```python
from build123d import *

# Parameters (mm, degrees)
F1_DEPTH = 20
F3_DEPTH = 20


with BuildPart() as f1:
    # F0 (on Top) → F1 (new body)
    with BuildSketch(Plane.XY):
        with BuildLine():
            ThreePointArc((-8.944425, -1.9), (0.955226, -9.093969), (9.144, 0))
            ThreePointArc((9.144, 0), (0.955226, 9.093969), (-8.944425, 1.9))
            ThreePointArc((-8.944425, 1.9), (-9.144, 0), (-8.944425, -1.9))
        make_face()
        with BuildLine():
            ThreePointArc((-8.944425, -1.9), (-9.144, 0), (-8.944425, 1.9))
            Line((-8.944425, 1.9), (-11.644, 1.9))
            Line((-11.644, 1.9), (-11.644, -1.9))
            Line((-11.644, -1.9), (-8.944425, -1.9))
        make_face()
    extrude(amount=F1_DEPTH)

    # F2 (on face) → F3 (cut, through all)
    with BuildSketch(Plane.XY.offset(20)):
        Polygon((6.6675, -3.849483), (6.6675, 3.849483), (0, 7.698966), (-6.6675, 3.849483), (-6.6675, -3.849483), (0, -7.698966), align=None)
    extrude(amount=-F3_DEPTH, mode=Mode.SUBTRACT)


solid = f1.part
```
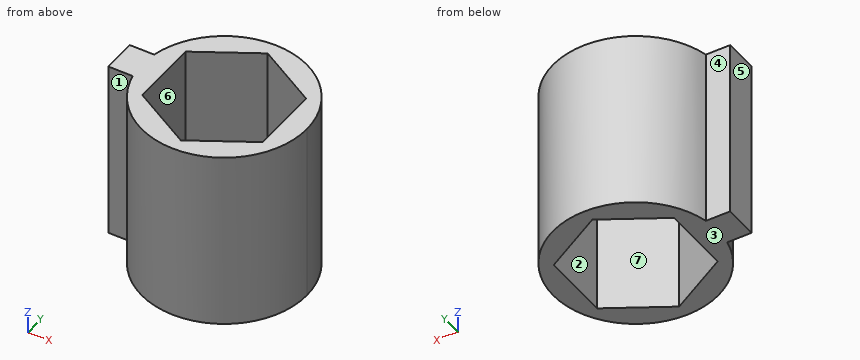
Check sheet for the modelled part. Datum: model origin and axes. Units: mm. Face numbers are marked on the shaded views. A direction names the side the tool comes from. Round coordinates to 2 decimals unless told otherwise and drop trailing zeros. Order: outer loops, then holes, each group sorted by start corner. A loop starts at its lowest first (then second) coordinate and runs counter-clockwise, first axis right, second up.
1) Section check C-C (x = -3). Record the boundary of the cut face in (y, z), and give its area (3 significant figures).
2) Section check D-D (x = -9.5). Record the boundary of the cut face in (y, z), and give its area (3 significant figures).
3) Section check B-B (y = 1.5). Record the boundary of the cut face in (x, z).
4) Mould release check, pull along X, two halves, no side actions. Record for the marked faces 4, 5, 6 and 7: +X half, -X half, draft (parallel to the pull), parting line (faces both ways), or undercut.
5) Scan lines: line 1 (X direction, y = 4.5, z = 3.75); line 2 (Y direction, x = -3, z = 8.75); line 3 (Y direction, x = 3.5, z = 17). Record each from-to range of solid material in increasing order.
6) Go/stop test with flat-tipped pins: pin 1 Ø6 at (y, z) = (-6, 17) entering from -X; pin 2 Ø1.5 at (x, z) = (-7.5, 11.5) entering from -Y; pin 3 Ø1.5 at (x, z) = (-5.5, 13) entering from +Y. Record where each tip stops, or that it passes through.
7) Section check A-A (z = 13.75). Record the boundary of the cut face in (x, y), and give its area (3 significant figures).
8) Tool access check on the marked faces 1, 2 and 3. Record the directions out of +Z, -Z, +X, -X, +Y, -Y that give a thin tool (end or side, any length) a straight path to the whole face; none if there is none.
Result:
1. outline: (-8.64, 0) - (-5.97, 0) - (-5.97, 20) - (-8.64, 20) - close; (5.97, 0) - (8.64, 0) - (8.64, 20) - (5.97, 20) - close
1. area: 107 mm2
2. outline: (-1.9, 0) - (1.9, 0) - (1.9, 20) - (-1.9, 20) - close
2. area: 76.0 mm2
3. outline: (-11.64, 0) - (-6.67, 0) - (-6.67, 20) - (-11.64, 20) - close; (6.67, 0) - (9.02, 0) - (9.02, 20) - (6.67, 20) - close
4. face 4: draft
4. face 5: -X half
4. face 6: undercut
4. face 7: undercut
5. line 1: x = -7.96 to -5.54, 5.54 to 7.96
5. line 2: y = -8.64 to -5.97, 5.97 to 8.64
5. line 3: y = -8.45 to -5.68, 5.68 to 8.45
6. pin 1: stops at x = -8.64
6. pin 2: stops at y = -6.17
6. pin 3: stops at y = 7.81
7. outline: (-11.64, -1.9) - (-8.94, -1.9) arc R9.14 ccw to (9.14, 0) arc R9.14 ccw to (-8.94, 1.9) - (-11.64, 1.9) - close; hole (-6.67, -3.85) - (0, -7.7) - (6.67, -3.85) - (6.67, 3.85) - (0, 7.7) - (-6.67, 3.85) - close
7. area: 118 mm2
8. face 1: +Z, -Z, -X, -Y
8. face 2: +Z, -Z
8. face 3: -Z, +X, -X, +Y, -Y
